Could you check a few things on this model? Use its own coordinates, in mm. A direction names the side the tool comes from. Give positions to 0.01 mm unless a question says otherwise; leave off trailing zeros. Order: outer loops, then holes, each group sorted by start corner. A loop starts at its lowest first (then second) coordinate and runs counter-clockwise, first axis right, second up. Notation, with made-up numbers: (-37.5, 74.25) -> (-3.5, 74.25) arc R19 cw to (-3.5, 88.25) -> close; hole circle Ø2 at (-0.5, 79.5). An arc over 180 degrees is marked (long way). Write each question's results on one line, items separated by ' | '.
```python
from build123d import *

# Parameters (mm, degrees)
F0_R     = 6.985
F1_DEPTH = 304.8
F3_D     = 5.7404
F3_DEPTH = 304.8
F3_TIP   = 1.7245901487
F5_D     = 5.08
F5_DEPTH = 25.4
F5_TIP   = 1.5261859723


with BuildPart() as f1:
    # F0 (on Front) → F1 (new body)
    with BuildSketch(Plane.XZ):
        Circle(F0_R)
    extrude(amount=F1_DEPTH)

    # F3
    with Locations(Plane(origin=(0, 0, 0), x_dir=(1, 0, 0), z_dir=(0, 1, 0))):
        with Locations((0, 0)):
            Hole(F3_D / 2, depth=F3_DEPTH)
            with Locations((0, 0, -(F3_DEPTH + F3_TIP / 2))):  # 118° drill point
                Cone(0, F3_D / 2, F3_TIP, mode=Mode.SUBTRACT)

    # F5 (one way)
    with BuildSketch(Plane(origin=(0, 0, 0), x_dir=(1, 0, 0), z_dir=(0, 0, -1))):
        with Locations((0, 76.1724114418)):
            Circle(F5_D / 2)
    extrude(amount=-F5_DEPTH, mode=Mode.SUBTRACT)
    with Locations(Plane(origin=(0, 0, 0), x_dir=(1, 0, 0), z_dir=(0, 0, -1))):
        with Locations((0, 76.1724114418)):
            with Locations((0, 0, -(F5_DEPTH + F5_TIP / 2))):  # 118° drill point
                Cone(0, F5_D / 2, F5_TIP, mode=Mode.SUBTRACT)


solid = f1.part
```
Q1. Thinking about a two-plate mould opening in Z: for faces 1 (the flat face through (3, 0, -1)), 2 (the cylindrical face through (-0.909, -150.266, 6.926)), 3 (the cylindrical face through (2.278, -154.534, 1.746)), which applies, +Z half, -Z half, draft (parallel to the pull), parting line (faces both ways), or undercut?
Here are the results:
face 1: draft | face 2: parting line | face 3: undercut
Q2. Suppose I cut it at A-A on x = 0. Please give me the cut outline in (y, z) (3 decimals), and give its area (3 significant figures).
Here are the results:
outline: (-304.8, -6.985) -> (0, -6.985) -> (0, -2.87) -> (-304.8, -2.87) -> close; (-304.8, 2.87) -> (-78.712, 2.87) -> (-78.712, 6.985) -> (-304.8, 6.985) -> close; (-73.632, 2.87) -> (0, 2.87) -> (0, 6.985) -> (-73.632, 6.985) -> close | area: 2,490 mm²
Q3. I'm going to push flat-ended pins straight in: pin 1 Ø3 at (x, y) = (2, -57) entering from +Z; pin 2 Ø4 at (x, y) = (0, -76.17) entering from +Z; pin 3 Ø6 at (x, y) = (5, -51.5) entering from +Z; pin 4 Ø8 at (x, z) = (5.5, 4.5) entering from +Y. Where does each tip first touch, or does it pass through?
Here are the results:
pin 1: stops at z = 6.97 | pin 2: stops at z = -2.06 | pin 3: stops at z = 6.69 | pin 4: stops at y = 0
Q4. Suppose I cut it at B-B on y = -39. Please give me the cut outline in (x, z) (3 decimals), and give its area (3 significant figures).
Here are the results:
outline: circle Ø13.97 at (0, 0); hole circle Ø5.74 at (0, 0) | area: 127 mm²
Q5. I need wall thicknesses on line 1 along Y through (x, z) = (0, 4.3); line 2 along X through (y, z) = (-50.5, -0.5); line 3 along Z through (x, y) = (0, -63) (3 decimals). Which ranges of each line are inside material? Lowest first, please.
Here are the results:
line 1: y = -304.8 to -78.71, -73.63 to 0 | line 2: x = -6.97 to -2.83, 2.83 to 6.97 | line 3: z = -6.985 to -2.87, 2.87 to 6.985
Q6. For faces 4 (the flat face through (3, -304.8, -1)), 5 (the cylindrical face through (-2.538, -76.284, 4.123)), which set-ups out of +Z, -Z, +X, -X, +Y, -Y let a thin tool reach every point of the face, with its end or its side?
Here are the results:
face 4: +Z, -Z, +X, -X, -Y | face 5: +Z
